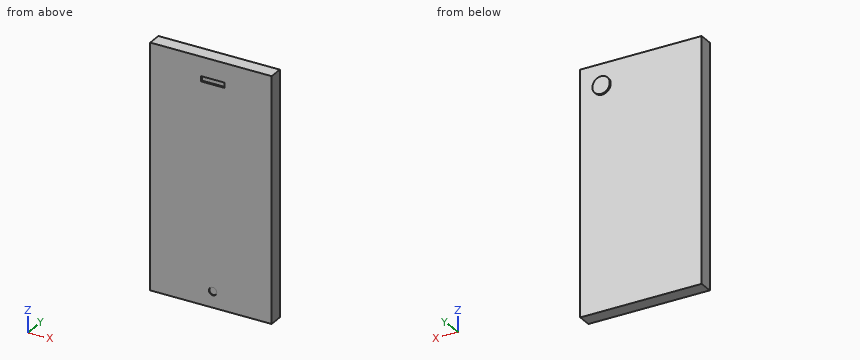
from build123d import *

# Parameters (mm, degrees)
F0_W     = 70
F0_H     = 140
F1_DEPTH = 8
F2_W     = 13.5
F2_H     = 3
F3_DEPTH = 1
F4_R     = 2.25
F5_DEPTH = 0.5
F6_R     = 5
F7_DEPTH = 1


# Not quite as in the source:
# - a feature of the source that left no trace in its solid (it failed there, or was rolled back) is left out


with BuildPart() as f1:
    # F0 (on Front) → F1 (new body)
    with BuildSketch(Plane.XZ):
        with Locations((5.7291688025, 19.6874958277)):
            Rectangle(F0_W, F0_H)
    extrude(amount=F1_DEPTH)

    # F2 (on face) → F3 (cut)
    with BuildSketch(Plane.XZ.offset(8)):
        with Locations((6.75, 77.1874958277)):
            Rectangle(F2_W, F2_H)
    extrude(amount=-F3_DEPTH, mode=Mode.SUBTRACT)

    # F4 (on face) → F5 (cut)
    with BuildSketch(Plane.XZ.offset(8)):
        with Locations((6.8374876864, -41.0625041723)):
            Circle(F4_R)
    extrude(amount=-F5_DEPTH, mode=Mode.SUBTRACT)

    # F6 (on face) → F7 (join)
    with BuildSketch(Plane(origin=(0, 0, 0), x_dir=(-1, 0, 0), z_dir=(0, 1, 0))):
        with Locations((-28.1465931075, 77.1049201327)):
            Circle(F6_R)
    extrude(amount=F7_DEPTH)


solid = f1.part
Input: part model. Units: mm. Frame: model coordinates. Give positions to 0.01 mm unless a question says otherwise; leave off trailing zeros. Order: outer loops, then holes, each group sorted by start corner. A loop starts at its lowest first (then second) coordinate and runs counter-clockwise, first axis right, second up. Notation, with made-up numbers: (-6, -11) - (6, -11) arc R18 ccw to (6, -7) - close; hole circle Ø5 at (52.25, -21.75). An arc over 180 degrees is marked (long way). Answer as a JSON object with one key per item and string values. Group by question number.
Q1. Line query: probe 1 along Y at (x, z) = (-10.5, 27.5). Output: solid intervals per line, ascending.
Q2. Cut plane B-B, the plane x = -4. Output: boundary loops of the cut face in (y, z), then the cut area to 3 significant figures.
Q3. Cut plane A-A, the plane z = -4.5. Output: boundary loops of the cut face in (x, y).
Q4. First-contact query: pin 1 Ø10 at (x, z) = (7, 49) entering from +Y. Flat tip, straight axial feed; report the tip coordinate or a pass-through.
Results:
{
 "1": {"probe 1": "-8 to 0"},
 "2": {"outline": "(-8, -50.31) - (0, -50.31) - (0, 89.69) - (-8, 89.69) - close", "area": "1,120 mm^2"},
 "3": {"outline": "(-29.27, -8) - (40.73, -8) - (40.73, 0) - (-29.27, 0) - close"},
 "4": {"pin 1": "y = 0"}
}
